Verification items for the finished model (mm, model axes). Give positions to 0.01 mm unless a question says otherwise; leave off trailing zeros. Order: outer loops, then holes, each group sorted by start corner. A loop starts at its lowest first (then second) coordinate and runs counter-clockwise, first axis right, second up. Notation, with made-up numbers: M 57,56 L 92,56 A18 ccw 92,68 Z; hole C 67.25,-25 d5. An arc over 180 degrees is marked long. Answer as a JSON object with one key per item and string values.
```python
from build123d import *

# Parameters (mm, degrees)
SKETCH_W     = 12.57
SKETCH_H     = 12.57
PAD_DEPTH    = 9.52
FILLET_R     = 0.7
SKETCH001_R  = 0.35
PAD001_DEPTH = 3.5


with BuildPart() as fillet_body:
    # Sketch → Pad (new body)
    with BuildSketch(Plane.XY.offset(0.1)):
        with Locations((4.76, 4.76)):
            Rectangle(SKETCH_W, SKETCH_H)
    extrude(amount=PAD_DEPTH)

    # Fillet
    fillet_edges = [fillet_body.edges().sort_by_distance(p)[0] for p in [
        (11.045, -1.525, 4.86),
        (11.045, 11.045, 4.86),
        (-1.525, -1.525, 4.86),
        (-1.525, 11.045, 4.86),
    ]]
    fillet(fillet_edges, radius=FILLET_R)


with BuildPart() as obj1:
    # Sketch001 → Pad001 (new body)
    with BuildSketch(Plane.XY.offset(0.5)):
        Circle(SKETCH001_R)
        with Locations((9.52, 9.52)):
            Circle(SKETCH001_R)
    extrude(amount=-PAD001_DEPTH)

    # obj1: union Fillet body
    add(fillet_body.part)


solid = obj1.part
```
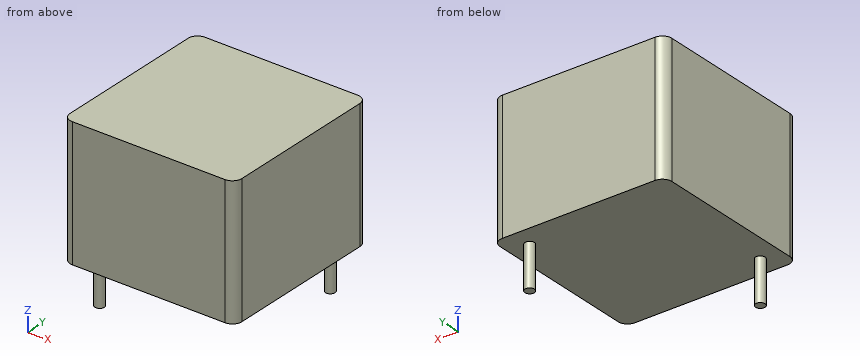
Q1. Section check B-B on x = 0. Record the cut outline in (y, z) (3 decimals).
Resolved:
{"outline": "M -1.525,0.1 L -0.35,0.1 L -0.35,-3 L 0.35,-3 L 0.35,0.1 L 11.045,0.1 L 11.045,9.62 L -1.525,9.62 Z"}
Q2. Section check A-A on z = -0.5. Record the cut outline in (x, y).
Resolved:
{"outline": "C 0,0 d0.7; C 9.52,9.52 d0.7"}
Q3. Section check C-C on y = 9.52. Record the cut outline in (x, z) (3 decimals), then the cut area to 3 significant figures.
Resolved:
{"outline": "M -1.525,0.1 L 9.17,0.1 L 9.17,-3 L 9.87,-3 L 9.87,0.1 L 11.045,0.1 L 11.045,9.62 L -1.525,9.62 Z", "area": "122 mm²"}
Q4. Gauge pin test, flat end, axial feed: pin 1 Ø6.5 at (x, y) = (3, 2.5) entering from -Z. Record the tip position at first contact, or that the pin passes through.
Resolved:
{"pin 1": "stops at z = 0.1"}
Q5. Section check D-D on y = 4. Record the cut outline in (x, z) (3 decimals), then the cut area to 3 significant figures.
Resolved:
{"outline": "M -1.525,0.1 L 11.045,0.1 L 11.045,9.62 L -1.525,9.62 Z", "area": "120 mm²"}
Q6. Material ranges on L1, parallel to Z at x = 1, y = 9; L2, parallel to Y at x = -1, z = 2.75, recorded low to high.
Resolved:
{"L1": "z = 0.1 to 9.62", "L2": "y = -1.5 to 11.02"}
